```python
from build123d import *

# Parameters (mm, degrees)
BOSS_EXTRUDE1_DEPTH = 1.5
SKETCH2_W           = 45
SKETCH2_H           = 5
SKETCH2_W_2         = 2.5
SKETCH2_H_2         = 20.5
SKETCH2_H_3         = 26
BOSS_EXTRUDE2_DEPTH = 10
SKETCH3_W           = 8.5
SKETCH3_H           = 15
BOSS_EXTRUDE3_DEPTH = 11
SKETCH4_W           = 11
SKETCH4_H           = 16
BOSS_EXTRUDE4_DEPTH = 11


with BuildPart() as part:
    # Sketch1 → Boss-Extrude1 (new body)
    with BuildSketch(Plane(origin=(0, 0, 0), x_dir=(1, 0, 0), z_dir=(0, 1, 0))):
        Polygon((-26, 48.5), (-14, 48.5), (-11, 52), (21, 52), (23, 50), (26, 50), (26, -50), (-26, -50), align=None)
    extrude(amount=BOSS_EXTRUDE1_DEPTH)

    # Sketch2 → Boss-Extrude2 (add)
    with BuildSketch(Plane(origin=(0, 1.5, 0), x_dir=(1, 0, 0), z_dir=(0, 1, 0))):
        with Locations((-2.5, 45.5)):
            Rectangle(SKETCH2_W, SKETCH2_H)
        with Locations((-23.75, 27.75)):
            Rectangle(SKETCH2_W_2, SKETCH2_H_2)
        with Locations((-23.75, 5.25)):
            Rectangle(SKETCH2_W_2, SKETCH2_H_2)
        with Locations((-23.75, -19)):
            Rectangle(SKETCH2_W_2, SKETCH2_H_3)
        with Locations((23.75, 10.25)):
            Rectangle(SKETCH2_W_2, SKETCH2_H_2)
        with Locations((23.75, 32.75)):
            Rectangle(SKETCH2_W_2, SKETCH2_H_2)
        with Locations((23.75, -12.25)):
            Rectangle(SKETCH2_W_2, SKETCH2_H_2)
    extrude(amount=BOSS_EXTRUDE2_DEPTH)

    # Sketch3 → Boss-Extrude3 (add)
    with BuildSketch(Plane(origin=(0, 1.5, 0), x_dir=(1, 0, 0), z_dir=(0, 1, 0))):
        with Locations((14.75, -47.5)):
            Rectangle(SKETCH3_W, SKETCH3_H)
    extrude(amount=BOSS_EXTRUDE3_DEPTH)

    # Sketch4 → Boss-Extrude4 (add)
    with BuildSketch(Plane(origin=(0, 1.5, 0), x_dir=(1, 0, 0), z_dir=(0, 1, 0))):
        with Locations((-14.5, -50)):
            Rectangle(SKETCH4_W, SKETCH4_H)
    extrude(amount=BOSS_EXTRUDE4_DEPTH)


solid = part.part
```
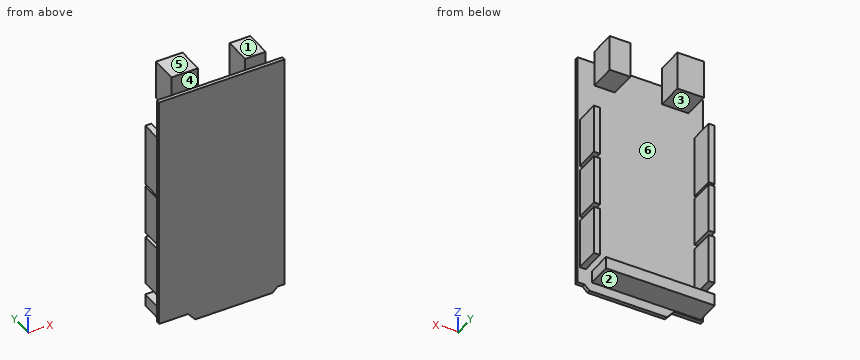
For this review, take the finished solid that the model builds, in its own axes (mm). Face numbers are marked on the shaded views. A direction names the side the tool comes from. Coordinates: 2 decimals unless noted, no trailing zeros. Order: outer loops, then holes, each group sorted by start corner. A loop starts at its lowest first (then second) coordinate and runs counter-clockwise, first axis right, second up. Notation, with made-up numbers: (-10.75, -6.5) -> (13.25, -6.5) arc R23 cw to (13.25, 3.5) -> close; hole circle Ø1 at (27.25, 56). An arc over 180 degrees is marked (long way). Use CSV: the item, a comma, the result in double quotes. Start each with the question number.
Item 1: For the marked faces 1, 2, 3 and 4, list the 3-axis set-ups (+Z, -Z, +X, -X, +Y, -Y) from which the entire face can be reached by the end or side of a thin tool; tool diameter is ignored.
Item 2: We need section C-C, the plane y = 8.75. Give the number of separate pieces and of enclosed holes in the cut face, then the cut area to 3 significant figures.
Item 3: Wall thickness on probe 1 along Z at (x, y) = (24, 10); probe 2 along Z at (x, y) = (-23, 10.25); probe 3 along X at (y, z) = (6, 22): over which ranges is each line inside the solid? List them lowest first.
Item 4: We need section A-A, the plane z = 4. Give the boundary of the cut face in (x, y).
Item 5: Insertion check: pin 1 (1.2 mm diameter, centred on x = 24.5, y = 4.5, fed in from -Z); pin 2 (5 mm diameter, centred on y = 6, z = -7.5, fed in from -X); pin 3 (3 mm diameter, centred on x = -8.5, y = 7.5, fed in from -Z). Each pin has a flat end and moves straight along its axis. Give the tip position at first contact, or say it passes through.
Item 6: We need section D-D, the plane x = -21. Give the boundary of the cut face in (y, z), then the cut area to 3 significant figures.
Item 7: We need section B-B, the plane x = 3. Give the boundary of the cut face in (y, z).
Item 8: Draft analysis for pull direction X (two halves, no side actions). For the marked faces 5 and 6, state which applies: pulls with the +X half, pulls with the -X half, needs draft (parallel to the pull), parting line crosses it, or undercut.
Derived:
1,face 1,"+Z, +X, +Y, -Y"
1,face 2,"-Z, +X, -X, +Y"
1,face 3,"-X, +Y"
1,face 4,"+Z, +X, -X, -Y"
2,separate pieces,"9"
2,enclosed holes,"0"
2,area,"850 mm^2"
3,probe 1,"z = -43 to -22.5, -20.5 to 0, 2 to 22.5"
3,probe 2,"z = -48 to -43, -38 to -17.5, -15.5 to 5, 6 to 32"
3,probe 3,"x = -25 to -22.5, 22.5 to 25"
4,outline,"(-26, 0) -> (26, 0) -> (26, 1.5) -> (25, 1.5) -> (25, 11.5) -> (22.5, 11.5) -> (22.5, 1.5) -> (-22.5, 1.5) -> (-22.5, 11.5) -> (-25, 11.5) -> (-25, 1.5) -> (-26, 1.5) -> close"
5,pin 1,"stops at z = -43"
5,pin 2,"stops at x = -25"
5,pin 3,"stops at z = -48"
6,outline,"(0, -48.5) -> (1.5, -48.5) -> (1.5, -48) -> (11.5, -48) -> (11.5, -43) -> (1.5, -43) -> (1.5, 50) -> (0, 50) -> close"
6,area,"198 mm^2"
7,outline,"(0, -52) -> (1.5, -52) -> (1.5, -48) -> (11.5, -48) -> (11.5, -43) -> (1.5, -43) -> (1.5, 50) -> (0, 50) -> close"
8,face 5,"needs draft"
8,face 6,"undercut"
